Can you work these out from the model? Positions are in its coordinate system, mm. Give positions to 0.01 mm unless a question says otherwise; leave off trailing zeros. Loops run counter-clockwise (first coordinate to the right, second up) from the corner with the lowest first, then second, coordinate; pieces in that order, holes last. Notation, with made-up numbers: (19, 4.5) - (47, 4.5) arc R31 cw to (47, 36.5) - close; hole circle Ø5 at (51.5, 57). An arc over 180 degrees is marked (long way). Use a Markdown table: item, result. Add a question column.
Autodesk Inventor part; units mm, degrees
ref_plane "YZ Plane" through (0, 0, 0) normal (1, 0, 0) x (0, 1, 0)
ref_plane "XZ Plane" through (0, 0, 0) normal (0, 1, 0) x (-1, 0, 0)
ref_plane "XY Plane" through (0, 0, 0) normal (0, 0, 1) x (1, 0, 0)
sketch "Sketch3" plane through (0, 0, 0) normal (1, 0, 0) x (0, 1, 0)
  line L0 (0, 0) -> (11.1125, 0)
  line L1 (11.1125, 0) -> (11.1125, -80)
  line L2 (11.1125, -80) -> (12.7, -80)
  line L3 (12.7, -80) -> (12.7, -1000)
  line L4 (12.7, -1000) -> (11.1125, -1000)
  line L5 (11.1125, -1000) -> (11.1125, -1080)
  line L6 (11.1125, -1080) -> (0, -1080)
  line L7 (0, 0) -> (0, -1080)
  dimension "d7" = 11.1125
  dimension "d8" = 80
  dimension "d9" = 1.5875
  dimension "d10" = 920
  dimension "d11" = 1.5875
  dimension "d12" = 80
  dimension "d13" = 11.1125
revolve "Revolution1" add sketch "Sketch3" angle 360 about axis through (0, 0, 0) along (0, 0, -1)
thread "Thread3"
thread "Thread4"
equation "\"d11\" = d9"
equation "\"d12\" = d8"
equation "\"d13\" = d7"
properties part number "Barra de deslizamiento"
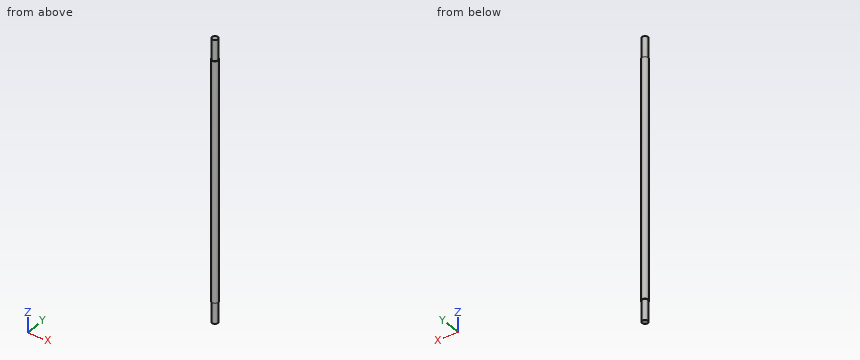
1. Suppose I cut it at A-A (x = 0). List the corners of the cut face in (y, z) for me, and give its area (3 significant figures).
2. Will these pins go through, and if not, where does the flat tip stop? P1, Ø12, axis at x = -10, z = -432.5, coming from the -Y side; P2, Ø4, axis at y = 2.5, z = -638.5, coming from the -X side; P3, Ø6, axis at y = 6.5, z = -191, coming from the -X side.
3. Please list where these lines run through material, in increasing order: line 1 along Y through (x, z) = (-6, -567); line 2 along X through (y, z) = (-0.5, -678.5); line 3 along Y through (x, z) = (-6.5, -237). Write a range as [from, to].
4. Suppose I cut it at C-C (z = -567). List the corners of the cut face in (x, y) for me, and give its area (3 significant figures).
Results below:
| question | item | result |
|---|---|---|
| 1 | outline | (-12.7, -1000) - (-11.11, -1000) - (-11.11, -1080) - (11.11, -1080) - (11.11, -1000) - (12.7, -1000) - (12.7, -80) - (11.11, -80) - (11.11, 0) - (-11.11, 0) - (-11.11, -80) - (-12.7, -80) - close |
| 1 | area | 26,900 mm² |
| 2 | P1 | y = -12.05 |
| 2 | P2 | x = -12.69 |
| 2 | P3 | x = -12.21 |
| 3 | line 1 | [-11.19, 11.19] |
| 3 | line 2 | [-12.69, 12.69] |
| 3 | line 3 | [-10.91, 10.91] |
| 4 | outline | circle Ø25.4 at (0, 0) |
| 4 | area | 507 mm² |
